Read the model definition and answer for the solid it produces. Units are mm, in the model's axes. A direction names the side the tool comes from. Coordinates: 2 decimals unless noted, no trailing zeros. Loops run counter-clockwise (first coordinate to the right, second up) from the corner with the lowest first, then second, coordinate; pieces in that order, holes last.
from build123d import *

# Parameters (mm, degrees)
SKETCH2_R           = 1.25
BOSS_EXTRUDE1_DEPTH = 12
SKETCH3_R           = 2.5
BOSS_EXTRUDE2_DEPTH = 1.5
FILLET1_R           = 1
SKETCH4_W           = 6.108207577
SKETCH4_H           = 1
CUT_EXTRUDE1_DEPTH  = 0.75


with BuildPart() as part:
    # Sketch2 → Boss-Extrude1 (new body)
    with BuildSketch(Plane.XY):
        Circle(SKETCH2_R)
    extrude(amount=-BOSS_EXTRUDE1_DEPTH)

    # Sketch3 → Boss-Extrude2 (add)
    with BuildSketch(Plane.XY):
        Circle(SKETCH3_R)
    extrude(amount=BOSS_EXTRUDE2_DEPTH)

    # Fillet1
    fillet1_edges = [part.edges().sort_by_distance(p)[0] for p in [
        (-2.5, 0, 1.5),
    ]]
    fillet(fillet1_edges, radius=FILLET1_R)

    # Sketch4 → Cut-Extrude1 (cut)
    with BuildSketch(Plane.XY.offset(1.5)):
        with Locations((-0.048809877, 0)):
            Rectangle(SKETCH4_W, SKETCH4_H)
    extrude(amount=-CUT_EXTRUDE1_DEPTH, mode=Mode.SUBTRACT)


solid = part.part
Item 1: A cutting plane is placed at A-A on x = 0. Determine the outline of the cut face in (y, z), then the cut area to 3 significant figures.
Numbers:
outline: (-2.5, 0) - (-1.25, 0) - (-1.25, -12) - (1.25, -12) - (1.25, 0) - (2.5, 0) - (2.5, 0.5) arc R1 ccw to (1.5, 1.5) - (0.5, 1.5) - (0.5, 0.75) - (-0.5, 0.75) - (-0.5, 1.5) - (-1.5, 1.5) arc R1 ccw to (-2.5, 0.5) - close
area: 36.3 mm2
Item 2: Given pin 1 (3 mm diameter, centred on x = 1.5, z = -7, fed in from +Y); pin 2 (0.6 mm diameter, centred on x = 1, z = 1, fed in from -Y); pin 3 (1.1 mm diameter, centred on x = 0, y = 0, fed in from +Z), each flat-ended and moving along its own axis, determine where each tip first touches the part or whether it passes through.
Numbers:
pin 1: stops at y = 1.25
pin 2: stops at y = -2.33
pin 3: stops at z = 1.5
Item 3: A cutting plane is placed at C-C on z = -7. Determine the outline of the cut face in (x, y), then the cut area to 3 significant figures.
Numbers:
outline: circle Ø2.5 at (0, 0)
area: 4.91 mm2
Item 4: A cutting plane is placed at B-B on y = 0. Determine the outline of the cut face in (x, z), then the cut area to 3 significant figures.
Numbers:
outline: (-2.5, 0) - (-1.25, 0) - (-1.25, -12) - (1.25, -12) - (1.25, 0) - (2.5, 0) - (2.5, 0.5) arc R1 ccw to (2.47, 0.75) - (-2.47, 0.75) arc R1 ccw to (-2.5, 0.5) - close
area: 33.7 mm2
Item 5: Which of the six approach directions +Z, -Z, +X, -X, +Y, -Y give full straight-line access (tool end or side, diameter ignored) to faces 1 (the face through (-1, -1, 0)), 2 (the face through (-0.54, -2.44, 0.25))?
Numbers:
face 1: -Z
face 2: +Z, -Z
Item 6: Find the intervals of material crossed by line 1 along Y through (x, z) = (0, -2.75); line 2 along Z through (x, y) = (0.55, -0.3); line 3 along Z through (x, y) = (0.75, -1.5), in increasing order.
Numbers:
line 1: y = -1.25 to 1.25
line 2: z = -12 to 0.75
line 3: z = 0 to 1.48
Item 7: Determine the mould class of faces 3 (the face through (0, 0, -12)), 4 (the face through (-0.27, -1.22, -5.92)), 5 (the face through (0, 0, 0.75)) for opening direction Y: released by +Y, released by -Y, zero draft, split by the parting line, or undercut.
Numbers:
face 3: zero draft
face 4: split by the parting line
face 5: undercut
